Here's how the part is built. I have some questions about the finished solid (model axes, mm). Give positions to 0.01 mm unless a question says otherwise; leave off trailing zeros. Loops run counter-clockwise (first coordinate to the right, second up) from the corner with the lowest first, then second, coordinate; pieces in that order, holes last.
Q1. I'm going to push flat-ended pins straight in: P1, Ø1.6, axis at y = 4, z = 336.5, coming from the +X side; P2, Ø3, axis at x = 0.5, z = 631, coming from the +Y side. Where does each tip first touch, or does it pass through?
Q2. Suppose I cut it at A-A (y = 1.25). Count the separate pieces of the cut face and the enclosed holes in it, and give its area (3 significant figures).
Q3. Suppose I cut it at B-B (z = 660.5). List the corners of the cut face in (x, y) for me.
Q4. I need wall thicknesses on probe 1 along Y at (x, z) = (-4, 226.5); probe 2 along X at (y, z) = (1.85, 225); probe 3 along X at (y, z) = (4.5, 169). Which ranges of each line are inside material? Lowest first, please.
Autodesk Inventor part; units mm, degrees
ref_plane "YZ Plane" through (0, 0, 0) normal (1, 0, 0) x (0, 1, 0)
ref_plane "XZ Plane" through (0, 0, 0) normal (0, 1, 0) x (-1, 0, 0)
ref_plane "XY Plane" through (0, 0, 0) normal (0, 0, 1) x (1, 0, 0)
sketch "Szkic1" plane through (0, 0, 0) normal (0, 0, 1) x (1, 0, 0)
  line L0 (0, 0) -> (4.5, 0)
  line L1 (4.5, 6.5) -> (-4.5, 6.5)
  line L2 (-4.5, 0) -> (4.5, 0)
  line L3 (4.5, 6.5) -> (4.5, 5)
  line L4 (4.5, 5) -> (3, 5)
  line L5 (3, 5) -> (3, 3.5)
  line L6 (3, 3.5) -> (4.5, 3.5)
  line L7 (-4.5, 6.5) -> (-4.5, 5)
  line L8 (-4.5, 5) -> (-3, 5)
  line L9 (-3, 5) -> (-3, 3.5)
  line L10 (-3, 3.5) -> (-4.5, 3.5)
  line L11 (-4.5, 6.5) -> (-4.5, 5)
  line L12 (-4.5, 3.5) -> (-4.5, 0)
  line L13 (4.5, 0) -> (4.5, 3.5)
  line L14 (4.5, 5) -> (4.5, 6.5)
  dimension "d1" = 6.5
  dimension "d2" = 9
  dimension "d3" = 1.5
  dimension "d4" = 1.5
  dimension "d5" = 1.5
  dimension "d6" = 1.5
  dimension "d7" = 1.5
  dimension "d8" = 1.5
extrude "Wyciągnięcie proste1" add sketch "Szkic1" along normal blind 900
sketch "Szkic2" plane through (-4.5, 6.5, 900) normal (0, 1, 0) x (1, 0, 0)
  line L0 (9, 900) -> (0, 900)
  line L1 (0, 900) -> (0, 0)
  line L2 (9, 0) -> (0, 0)
  line L3 (9, 900) -> (9, 0)
  line L4 (0, 0) -> (4.5, 0)
  line L5 (9, 0) -> (0, 0)
  line L6 (4.5, 0) -> (4.5, 900)
  line L7 (4.5, 900) -> (4.5, 855)
  circle A0 centre (4.5, 855) radius 1.75
  dimension "d11" = 4.5
  dimension "d12" = 45
  dimension "d13" = 3.5
extrude "Wyciągnięcie proste2" cut sketch "Szkic2" against normal up to next contours A0 L6 | L6 A0
sketch "Szkic3" plane through (-4.5, 6.5, 900) normal (0, 1, 0) x (1, 0, 0)
  circle A0 centre (4.5, 855) radius 1.75
  circle A1 centre (4.5, 855) radius 3
  point P0 (4.5, 900)
  dimension "d16" = 6
extrude "Wyciągnięcie proste3" cut sketch "Szkic3" against normal blind 4
pattern_linear "Szyk prostokątny1" count 19 spacing 45 along (0, 0, 1) of "Wyciągnięcie proste3"
pattern_linear "Szyk prostokątny2" count 19 spacing 45 along (0, 0, 1) of "Wyciągnięcie proste2"
properties part number "Prowadnica liniowa MGN9R 900mm"
Solutions:
1. P1: stops at x = 4.5
1. P2: stops at y = 2.5
2. separate pieces: 1
2. enclosed holes: 19
2. area: 7,920 mm2
3. outline: (-4.5, 0) - (4.5, 0) - (4.5, 3.5) - (3, 3.5) - (3, 5) - (4.5, 5) - (4.5, 6.5) - (-4.5, 6.5) - (-4.5, 5) - (-3, 5) - (-3, 3.5) - (-4.5, 3.5) - close
4. probe 1: y = 0 to 3.5, 5 to 6.5
4. probe 2: x = -4.5 to -1.75, 1.75 to 4.5
4. probe 3: x = -3 to 3
